from build123d import *

# Parameters (mm, degrees)
SKETCH1_W               = 100
SKETCH1_H               = 60
BOSS_EXTRUDE1_DEPTH     = 55
CUT_EXTRUDE1_START      = -30
SKETCH2_W               = 80
SKETCH2_H               = 100
CUT_EXTRUDE1_DEPTH      = 45
CUT_EXTRUDE2_DEPTH      = 81.156097709
CUT_EXTRUDE2_DEPTH_BACK = 81.156097709
SKETCH3_R               = 1.75
CUT_EXTRUDE3_START      = 55
CUT_EXTRUDE3_DEPTH      = 52
BOSS_EXTRUDE2_START     = 15
SKETCH5_W               = 3
SKETCH5_H               = 20
BOSS_EXTRUDE2_DEPTH     = 45
CHAMFER1_SIZE           = 3
CUT_EXTRUDE4_DEPTH      = 81.156097709
CUT_EXTRUDE4_DEPTH_BACK = 81.156097709
SKETCH6_R               = 1.75
CUT_EXTRUDE5_START      = 30
SKETCH7_R               = 3
CUT_EXTRUDE5_DEPTH      = 5
BOSS_EXTRUDE3_START     = 50
SKETCH8_W               = 10
SKETCH8_H               = 5
BOSS_EXTRUDE3_DEPTH     = 5
BOSS_EXTRUDE4_START     = -50
SKETCH8_2_W             = 10
SKETCH8_2_H             = 5
BOSS_EXTRUDE4_DEPTH     = 5
BOSS_EXTRUDE5_START     = 30
SKETCH9_W               = 10
SKETCH9_H               = 5
BOSS_EXTRUDE5_DEPTH     = 5


# Some blends are built 0.0001 mm under size
with BuildPart() as part:
    # Sketch1 → Boss-Extrude1 (new body)
    with BuildSketch(Plane(origin=(0, 0, 0), x_dir=(1, 0, 0), z_dir=(0, 1, 0))):
        Rectangle(SKETCH1_W, SKETCH1_H)
    extrude(amount=BOSS_EXTRUDE1_DEPTH)

    # Sketch2 → Cut-Extrude1 (cut)
    with BuildSketch(Plane.XY.offset(CUT_EXTRUDE1_START)):
        Rectangle(SKETCH2_W, SKETCH2_H)
    extrude(amount=CUT_EXTRUDE1_DEPTH, mode=Mode.SUBTRACT)

    # Sketch3 → Cut-Extrude2 (cut, two sides: drawn at the far end of the back side and taken through both)
    with BuildSketch(Plane(origin=(0, 0, 0), x_dir=(1, 0, 0), z_dir=(0, 1, 0)).offset(-CUT_EXTRUDE2_DEPTH_BACK)):
        with Locations(Location((-45, 15, 0), (0, 0, 90))):
            Circle(SKETCH3_R)
        with Locations(Location((45, 15, 0), (0, 0, 90))):
            Circle(SKETCH3_R)
        with Locations(Location((45, -20, 0), (0, 0, 90))):
            Circle(SKETCH3_R)
        with Locations(Location((-45, -20, 0), (0, 0, 90))):
            Circle(SKETCH3_R)
    extrude(amount=CUT_EXTRUDE2_DEPTH + CUT_EXTRUDE2_DEPTH_BACK, mode=Mode.SUBTRACT)

    # Sketch4 → Cut-Extrude3 (cut)
    with BuildSketch(Plane(origin=(0, 0, 0), x_dir=(1, 0, 0), z_dir=(0, 1, 0)).offset(CUT_EXTRUDE3_START)):
        Polygon((44.159672203, -23.360632261), (47.490229012, -22.408061351), (48.330556809, -19.04742909), (45.840327797, -16.639367739), (42.509770988, -17.591938649), (41.669443191, -20.95257091), align=None)
        Polygon((44.794589767, 18.458006165), (41.902573698, 16.551112602), (42.107983932, 13.093106437), (45.205410233, 11.541993835), (48.097426302, 13.448887398), (47.892016068, 16.906893563), align=None)
        Polygon((-45.840327797, -23.360632261), (-42.509770988, -22.408061351), (-41.669443191, -19.04742909), (-44.159672203, -16.639367739), (-47.490229012, -17.591938649), (-48.330556809, -20.95257091), align=None)
        Polygon((-45.205410233, 18.458006165), (-48.097426302, 16.551112602), (-47.892016068, 13.093106437), (-44.794589767, 11.541993835), (-41.902573698, 13.448887398), (-42.107983932, 16.906893563), align=None)
    extrude(amount=-CUT_EXTRUDE3_DEPTH, mode=Mode.SUBTRACT)

    # Sketch5 → Boss-Extrude2 (add)
    with BuildSketch(Plane.XY.offset(BOSS_EXTRUDE2_START)):
        with Locations((-38.5, 25)):
            Rectangle(SKETCH5_W, SKETCH5_H)
        with Locations((38.5, 25)):
            Rectangle(SKETCH5_W, SKETCH5_H)
    extrude(amount=-BOSS_EXTRUDE2_DEPTH)

    # Chamfer1
    chamfer1_edges = [part.edges().sort_by_distance(p)[0] for p in [
        (37, 15, -7.5),
        (37, 35, -7.5),
        (-37, 15, -7.5),
        (-37, 35, -7.5),
    ]]
    chamfer(chamfer1_edges, length=CHAMFER1_SIZE - 0.0001)  # a hair under: the kernel refuses the full size

    # Sketch6 → Cut-Extrude4 (cut, two sides: drawn at the far end of the back side and taken through both)
    with BuildSketch(Plane.XY.offset(-CUT_EXTRUDE4_DEPTH_BACK)):
        with Locations((32, 25)):
            Circle(SKETCH6_R)
        with Locations((-32, 25)):
            Circle(SKETCH6_R)
    extrude(amount=CUT_EXTRUDE4_DEPTH + CUT_EXTRUDE4_DEPTH_BACK, mode=Mode.SUBTRACT)

    # Sketch7 → Cut-Extrude5 (cut)
    with BuildSketch(Plane.XY.offset(CUT_EXTRUDE5_START)):
        with Locations(Location((-32, 25, 0), (0, 0, 180))):
            Circle(SKETCH7_R)
        with Locations(Location((32, 25, 0), (0, 0, 180))):
            Circle(SKETCH7_R)
    extrude(amount=-CUT_EXTRUDE5_DEPTH, mode=Mode.SUBTRACT)

    # Sketch8 → Boss-Extrude3 (add)
    with BuildSketch(Plane(origin=(0, 0, 0), x_dir=(0, 0, -1), z_dir=(1, 0, 0)).offset(BOSS_EXTRUDE3_START)):
        with Locations((0, -2.5)):
            Rectangle(SKETCH8_W, SKETCH8_H)
    extrude(amount=-BOSS_EXTRUDE3_DEPTH)

    # Sketch8<2> → Boss-Extrude4 (add)
    with BuildSketch(Plane(origin=(0, 0, 0), x_dir=(0, 0, -1), z_dir=(1, 0, 0)).offset(BOSS_EXTRUDE4_START)):
        with Locations((0, -2.5)):
            Rectangle(SKETCH8_2_W, SKETCH8_2_H)
    extrude(amount=BOSS_EXTRUDE4_DEPTH)

    # Sketch9 → Boss-Extrude5 (add)
    with BuildSketch(Plane.XY.offset(BOSS_EXTRUDE5_START)):
        with Locations((0, -2.5)):
            Rectangle(SKETCH9_W, SKETCH9_H)
    extrude(amount=-BOSS_EXTRUDE5_DEPTH)

    # Chamfer2
    # the kernel refuses this chamfer: 5 mm, written as the material it takes off along each edge
    with BuildSketch(Plane(origin=(-46.666666667, 51.666666667, -26.666666667), x_dir=(0, 0.7071067811865475, 0.7071067811865475), z_dir=(-0.5773502691896257, 0.5773502691896257, -0.5773502691896257)), Plane(origin=(46.666666667, 51.666666667, 26.666666667), x_dir=(0, 0.7071067811865475, -0.7071067811865475), z_dir=(0.5773502691896257, 0.5773502691896257, 0.5773502691896257))) as chamfer2_piece_1:
        Polygon((-3.535533906, 2.041241452), (3.535533906, 2.041241452), (0, -4.082482905), align=None)
    extrude(amount=6.350852961, mode=Mode.SUBTRACT)
    with BuildSketch(Plane(origin=(46.666666667, 51.666666667, -26.666666667), x_dir=(0, 0.7071067811865475, 0.7071067811865475), z_dir=(0.577350269189626, 0.5773502691896256, -0.5773502691896256)), Plane(origin=(-46.666666667, 51.666666667, 26.666666667), x_dir=(0, 0.7071067811865475, -0.7071067811865475), z_dir=(-0.577350269189626, 0.5773502691896256, 0.5773502691896256))) as chamfer2_piece_2:
        Polygon((-3.535533906, -2.041241452), (3.535533906, -2.041241452), (0, 4.082482905), align=None)
    extrude(amount=6.350852961, mode=Mode.SUBTRACT)
    with BuildSketch(Plane(origin=(-50, -12.85841494, -30), x_dir=(0.9996219169112968, 0, -0.027495876610586317), z_dir=(0, 1, 0)), Plane(origin=(-50, -12.85841494, 30), x_dir=(-0.027495876610586317, 0, -0.9996219169112968), z_dir=(0, 1, 0))) as chamfer2_piece_3:
        with BuildLine():
            Line((5.143365976, 0), (-0.282735774, -5.135588968))
            Line((-0.282735774, -5.135588968), (-0.382697966, -5.13283938))
            ThreePointArc((-0.382697966, -5.13283938), (-0.170646135, -2.566989148), (-0.099962192, 0.002749588))
            Line((-0.099962192, 0.002749588), (0.002749588, 0.099962192))
            ThreePointArc((0.002749588, 0.099962192), (2.572488324, 0.029278248), (5.146115564, 0.099962192))
            Line((5.146115564, 0.099962192), (5.143365976, 0))
        make_face()
    extrude(amount=80.71682988, mode=Mode.SUBTRACT)
    with BuildSketch(Plane(origin=(50, -12.85841494, -30), x_dir=(-0.9996219169112968, 0, -0.027495876610586317), z_dir=(0, 1, 0)), Plane(origin=(50, -12.85841494, 30), x_dir=(0.027495876610586317, 0, -0.9996219169112968), z_dir=(0, 1, 0))) as chamfer2_piece_4:
        with BuildLine():
            Line((5.143365976, 0), (-0.282735774, 5.135588968))
            Line((-0.282735774, 5.135588968), (-0.382697966, 5.13283938))
            ThreePointArc((-0.382697966, 5.13283938), (-0.170646135, 2.566989148), (-0.099962192, -0.002749588))
            Line((-0.099962192, -0.002749588), (0.002749588, -0.099962192))
            ThreePointArc((0.002749588, -0.099962192), (2.572488324, -0.029278248), (5.146115564, -0.099962192))
            Line((5.146115564, -0.099962192), (5.143365976, 0))
        make_face()
    extrude(amount=80.71682988, mode=Mode.SUBTRACT)
    with BuildSketch(Plane(origin=(50, 55, 42.85841494), x_dir=(-0.9996219169112968, 0.027495876610586317, 0), z_dir=(0, 0, -1))) as chamfer2_piece_5:
        with BuildLine():
            Line((5.143365976, 0), (-0.282735774, -5.135588968))
            Line((-0.282735774, -5.135588968), (-0.382697966, -5.13283938))
            ThreePointArc((-0.382697966, -5.13283938), (-0.170646135, -2.566989148), (-0.099962192, 0.002749588))
            Line((-0.099962192, 0.002749588), (0.002749588, 0.099962192))
            ThreePointArc((0.002749588, 0.099962192), (2.572488324, 0.029278248), (5.146115564, 0.099962192))
            Line((5.146115564, 0.099962192), (5.143365976, 0))
        make_face()
    extrude(amount=85.71682988, mode=Mode.SUBTRACT)
    with BuildSketch(Plane(origin=(-50, 55, -42.85841494), x_dir=(-0.027495876610586317, -0.9996219169112968, 0), z_dir=(0, 0, 1))) as chamfer2_piece_6:
        with BuildLine():
            Line((5.143365976, 0), (-0.282735774, 5.135588968))
            Line((-0.282735774, 5.135588968), (-0.382697966, 5.13283938))
            ThreePointArc((-0.382697966, 5.13283938), (-0.170646135, 2.566989148), (-0.099962192, -0.002749588))
            Line((-0.099962192, -0.002749588), (0.002749588, -0.099962192))
            ThreePointArc((0.002749588, -0.099962192), (2.572488324, -0.029278248), (5.146115564, -0.099962192))
            Line((5.146115564, -0.099962192), (5.143365976, 0))
        make_face()
    extrude(amount=85.71682988, mode=Mode.SUBTRACT)
    with BuildSketch(Plane(origin=(-62.85841494, 55, 30), x_dir=(0, 0.027495876610586317, -0.9996219169112968), z_dir=(1, 0, 0))) as chamfer2_piece_7:
        with BuildLine():
            Line((5.143365976, 0), (-0.282735774, -5.135588968))
            Line((-0.282735774, -5.135588968), (-0.382697966, -5.13283938))
            ThreePointArc((-0.382697966, -5.13283938), (-0.170646135, -2.566989148), (-0.099962192, 0.002749588))
            Line((-0.099962192, 0.002749588), (0.002749588, 0.099962192))
            ThreePointArc((0.002749588, 0.099962192), (2.572488324, 0.029278248), (5.146115564, 0.099962192))
            Line((5.146115564, 0.099962192), (5.143365976, 0))
        make_face()
    extrude(amount=125.71682988, mode=Mode.SUBTRACT)
    with BuildSketch(Plane(origin=(62.85841494, 55, -30), x_dir=(0, -0.9996219169112968, -0.027495876610586317), z_dir=(-1, 0, 0))) as chamfer2_piece_8:
        with BuildLine():
            Line((5.143365976, 0), (-0.282735774, 5.135588968))
            Line((-0.282735774, 5.135588968), (-0.382697966, 5.13283938))
            ThreePointArc((-0.382697966, 5.13283938), (-0.170646135, 2.566989148), (-0.099962192, -0.002749588))
            Line((-0.099962192, -0.002749588), (0.002749588, -0.099962192))
            ThreePointArc((0.002749588, -0.099962192), (2.572488324, -0.029278248), (5.146115564, -0.099962192))
            Line((5.146115564, -0.099962192), (5.143365976, 0))
        make_face()
    extrude(amount=125.71682988, mode=Mode.SUBTRACT)


solid = part.part
Design review of the part built by this model. Coordinates are the model's own, in mm. A direction names the side the tool comes from. Coordinates: 2 decimals unless noted, no trailing zeros. Order: outer loops, then holes, each group sorted by start corner. A loop starts at its lowest first (then second) coordinate and runs counter-clockwise, first axis right, second up. Notation, with made-up numbers: (87, 70) - (138, 70) arc R30 cw to (138, 106) - close; hole circle Ø9 at (12, 44.25). An arc over 180 degrees is marked (long way). Put each result on its own line as item: value.
1) Take a section at A-A, the plane x = -32. Give the boundary of the cut face in (y, z), and give its area (3 significant figures).
Response values:
outline: (0, 15) - (23.25, 15) - (23.25, 25) - (22, 25) - (22, 30) - (0, 30) - close; (26.75, 15) - (50, 15) - (50, -30) - (55, -25) - (55, 25) - (50, 30) - (28, 30) - (28, 25) - (26.75, 25) - close
area: 960 mm²
2) Take a section at C-C, the plane x = 23.5. Give the boundary of the cut face in (y, z), and give its area (4 significant figures).
Response values:
outline: (0, 15) - (50, 15) - (50, -30) - (55, -25) - (55, 25) - (50, 30) - (0, 30) - close
area: 1,025 mm²
3) The part is to be moulded in two halves that separate along Z. For faces 1 (the face through (-48, 25, 27)), 2 (the face through (-43.29, 1.48, 20.38)), 3 (the face through (38, 17, -7)), 4 (the face through (-48, -3, -5)), say which applies: released by +Z, released by -Z, zero draft, split by the parting line, or undercut.
Response values:
face 1: released by +Z
face 2: undercut
face 3: zero draft
face 4: released by -Z
4) Tool access review of faces 5 (the face through (37, 25, -7)), 6 (the face through (-43.7, 3, -13.5)), 7 (the face through (50, 22, 0)): name each direction out of +Z, -Z, +X, -X, +Y, -Y from which nothing blocks a thin tool from reaching the whole face with its end or side.
Response values:
face 5: -Z, -Y
face 6: +Y
face 7: +Z, -Z, +X, +Y, -Y
5) Insertion check: P1, Ø4, axis at y = -3, z = 27, coming from the +X side; P2, Ø12, axis at x = -1.5, z = 8, coming from the -Y side; P3, Ø2, axis at x = 32, y = 25, coming from the +Z side; P4, Ø5.5, axis at x = 44, z = 20, coming from the +Y side. Each pin has a flat end and moves straight along its axis. Give the tip position at first contact, or say it passes through.
Response values:
P1: stops at x = 5
P2: stops at y = 50
P3: passes through
P4: stops at y = 55
6) Wall thickness on L1, parallel to X at y = 1.3, z = -15; L2, parallel to X at y = 39.5, z = -3.5; L3, parallel to Z at x = -26, y = 18: over which ranges is each line inside the solid? List them lowest first. Write a range as from..to.
Response values:
L1: x = -50..-46.75, -43.25..-40, 40..43.25, 46.75..50
L2: x = -50..-40, 40..50
L3: z = 15..30
7) Take a section at B-B, the plane y = 25. Count the separate pieces of the cut face and the enclosed holes in it, and give its area (3 significant figures).
Response values:
separate pieces: 3
enclosed holes: 4
area: 2,370 mm²
